Model file for the job. Use its own axes, mm. Face numbers are marked on the shaded views. Coordinates: 2 decimals unless noted, no trailing zeros. Write each loop counter-clockwise with the first axis right and the second up, starting at its lowest first coordinate (ties: lowest second). Pieces come first, ordered by that corner, then holes.
Q1. Pull direction Z, two halves, no side cores. Call the marked faces 1 and 2: released by +Z, released by -Z, zero draft, split by the parting line, or undercut.
Q2. Band-saw the part on C-C, the plane x = 46. Write the cut outline in (y, z), plus the area to 3 significant figures.
Q3. Drill centre lines: probe 1 along Z at (x, y) = (26, -1.55); probe 2 along Z at (x, y) = (-50, 0.8); probe 3 along Z at (x, y) = (58.4, 1.6). Where is each one in solid material? Low to high.
Q4. Pin check, flat tips, straight feed: P1, Ø1.1, axis at y = 1, z = 6.5, coming from the -X side; P2, Ø3, axis at x = 15.5, y = 2.5, coming from the -Z side; P3, Ø1, axis at x = -24, y = 1, coming from the +Z side. Stop position of each tip, or through.
Q5. Band-saw the part on D-D, the plane z = 2.1. Write the cut outline in (x, y).
Q6. Band-saw the part on A-A, the plane z = 9.2. Write the cut outline in (x, y), plus the area to 3 significant figures.
Q7. Band-saw the part on B-B, the plane x = -38. Write the cut outline in (y, z), plus the area to 3 significant figures.
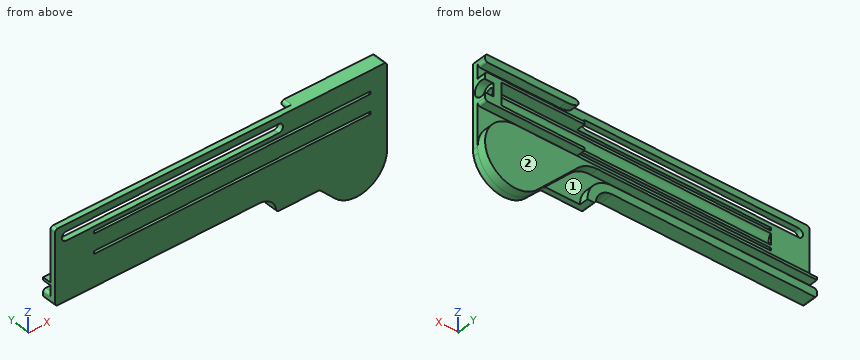
from build123d import *

# Parameters (mm, degrees)
BOSS_EXTRUDE2_DEPTH = 2
BOSS_EXTRUDE3_DEPTH = 3.2
BOSS_EXTRUDE4_START = 3.2
BOSS_EXTRUDE4_DEPTH = 3.2
SKETCH9_W           = 10
SKETCH9_H           = 3.2
BOSS_EXTRUDE5_DEPTH = 6
SKETCH8_R           = 2.8
CUT_EXTRUDE1_DEPTH  = 3.1
SKETCH10_R          = 1.4
CUT_EXTRUDE2_DEPTH  = 121.272440734
SKETCH11_R          = 2.55
CUT_EXTRUDE3_DEPTH  = 100
SKETCH12_W          = 30
SKETCH12_H          = 1
BOSS_EXTRUDE6_DEPTH = 3.2
SKETCH13_W          = 100
SKETCH13_H          = 1
CUT_EXTRUDE4_DEPTH  = 67.33136513
BOSS_EXTRUDE7_DEPTH = 3.2
CUT_EXTRUDE5_DEPTH  = 67.33136513
FILLET1_R           = 10
BOSS_EXTRUDE8_START = 2
BOSS_EXTRUDE8_DEPTH = 2
CUT_EXTRUDE6_DEPTH  = 67.33136513
FILLET2_R           = 1


with BuildPart() as part:
    # Sketch4 → Boss-Extrude2 (new body)
    with BuildSketch(Plane(origin=(0, 0, 0), x_dir=(1, 0, 0), z_dir=(0, 1, 0))):
        with BuildLine():
            Line((-60, -13.3), (60, -13.3))
            Line((60, -13.3), (60, 19.3))
            Line((60, 19.3), (20, 19.3))
            ThreePointArc((20, 19.3), (18.242640687, 15.057359313), (14, 13.3))
            Line((14, 13.3), (-60, 13.3))
            Line((-60, 13.3), (-60, -13.3))
        make_face()
    extrude(amount=-BOSS_EXTRUDE2_DEPTH)

    # Sketch5 → Boss-Extrude3 (add)
    with BuildSketch(Plane(origin=(0, 0, 0), x_dir=(1, 0, 0), z_dir=(0, 1, 0))):
        with BuildLine():
            Line((23.443650814, 7.1), (41.221825407, 24.878174593))
            ThreePointArc((41.221825407, 24.878174593), (59.162674858, 21.309517756), (49, 6.1))
            Line((49, 6.1), (-60, 6.1))
            Line((-60, 6.1), (-60, 7.1))
            Line((-60, 7.1), (23.443650814, 7.1))
        make_face()
    extrude(amount=BOSS_EXTRUDE3_DEPTH)

    # Sketch6 → Boss-Extrude4 (add)
    with BuildSketch(Plane(origin=(0, 0, 0), x_dir=(1, 0, 0), z_dir=(0, 1, 0)).offset(BOSS_EXTRUDE4_START)):
        with BuildLine():
            Line((-60, 10.3), (14, 10.3))
            ThreePointArc((14, 10.3), (20.363961031, 12.936038969), (23, 19.3))
            Line((23, 19.3), (20, 19.3))
            ThreePointArc((20, 19.3), (18.242640687, 15.057359313), (14, 13.3))
            Line((14, 13.3), (-60, 13.3))
            Line((-60, 13.3), (-60, 10.3))
        make_face()
    extrude(amount=-BOSS_EXTRUDE4_DEPTH)

    # Sketch9 → Boss-Extrude5 (add)
    with BuildSketch(Plane(origin=(60, 0, 0), x_dir=(0, 0, -1), z_dir=(1, 0, 0))):
        with Locations((-2.1, 1.6)):
            Rectangle(SKETCH9_W, SKETCH9_H)
    extrude(amount=-BOSS_EXTRUDE5_DEPTH)

    # Sketch8 → Cut-Extrude1 (cut)
    with BuildSketch(Plane(origin=(60, 0, 0), x_dir=(0, 0, -1), z_dir=(1, 0, 0))):
        with Locations((-2.1, 1.6)):
            Circle(SKETCH8_R)
    extrude(amount=-CUT_EXTRUDE1_DEPTH, mode=Mode.SUBTRACT)

    # Sketch10 → Cut-Extrude2 (cut, through all)
    with BuildSketch(Plane(origin=(56.9, 0, 0), x_dir=(0, 0, -1), z_dir=(1, 0, 0))):
        with Locations((-2.1, 1.6)):
            Circle(SKETCH10_R)
    extrude(amount=-CUT_EXTRUDE2_DEPTH, mode=Mode.SUBTRACT)

    # Sketch11 → Cut-Extrude3 (cut)
    with BuildSketch(Plane.ZY.offset(-54)):
        with Locations((2.1, 1.6)):
            Circle(SKETCH11_R)
    extrude(amount=CUT_EXTRUDE3_DEPTH, mode=Mode.SUBTRACT)

    # Sketch12 → Boss-Extrude6 (add)
    with BuildSketch(Plane(origin=(0, 0, 0), x_dir=(1, 0, 0), z_dir=(0, 1, 0))):
        with Locations((39, 2.4)):
            Rectangle(SKETCH12_W, SKETCH12_H)
    boss_extrude6 = extrude(amount=BOSS_EXTRUDE6_DEPTH)

    # Sketch13 → Cut-Extrude4 (cut, through all)
    with BuildSketch(Plane(origin=(0, 0, 0), x_dir=(1, 0, 0), z_dir=(0, 1, 0))):
        with Locations((4, 1.4)):
            Rectangle(SKETCH13_W, SKETCH13_H)
    cut_extrude4 = extrude(amount=-CUT_EXTRUDE4_DEPTH, mode=Mode.SUBTRACT)

    # Mirror1: Boss-Extrude6, Cut-Extrude4 across plane
    add(boss_extrude6.mirror(Plane.XY.offset(2.1)))
    add(cut_extrude4.mirror(Plane.XY.offset(2.1)), mode=Mode.SUBTRACT)

    # Sketch14 → Boss-Extrude7 (add)
    with BuildSketch(Plane(origin=(0, 0, 0), x_dir=(1, 0, 0), z_dir=(0, 1, 0))):
        with BuildLine():
            Line((60, -10.6), (30.518376618, -10.6))
            ThreePointArc((30.518376618, -10.6), (26.990656613, -11.301707138), (24, -13.3))
            Line((24, -13.3), (60, -13.3))
            Line((60, -13.3), (60, -10.6))
        make_face()
    extrude(amount=BOSS_EXTRUDE7_DEPTH)

    # Sketch15 → Cut-Extrude5 (cut, through all)
    with BuildSketch(Plane(origin=(0, 0, 0), x_dir=(1, 0, 0), z_dir=(0, 1, 0))):
        with BuildLine():
            Line((-56, -7.6), (20.8, -7.6))
            ThreePointArc((20.8, -7.6), (22.4, -9.2), (20.8, -10.8))
            Line((20.8, -10.8), (-56, -10.8))
            ThreePointArc((-56, -10.8), (-57.6, -9.2), (-56, -7.6))
        make_face()
    extrude(amount=-CUT_EXTRUDE5_DEPTH, mode=Mode.SUBTRACT)

    # Fillet1
    fillet1_edges = [part.edges().sort_by_distance(p)[0] for p in [
        (23.443650814, 1.6, -7.1),
    ]]
    fillet(fillet1_edges, radius=FILLET1_R)

    # Sketch16 → Boss-Extrude8 (add)
    with BuildSketch(Plane.XZ.offset(BOSS_EXTRUDE8_START)):
        with BuildLine():
            Line((59.777754868, -19.3), (35.643650814, -19.3))
            Line((35.643650814, -19.3), (41.221825407, -24.878174593))
            ThreePointArc((41.221825407, -24.878174593), (52.166761501, -27.634306887), (59.777754868, -19.3))
        make_face()
    extrude(amount=-BOSS_EXTRUDE8_DEPTH)

    # Sketch17 → Cut-Extrude6 (cut, through all)
    with BuildSketch(Plane(origin=(0, 0, 0), x_dir=(1, 0, 0), z_dir=(0, 1, 0))):
        with BuildLine():
            Line((60, 17.1), (60, 19.3))
            Line((60, 19.3), (59.777754868, 19.3))
            ThreePointArc((59.777754868, 19.3), (59.944297683, 18.205598582), (60, 17.1))
        make_face()
    extrude(amount=-CUT_EXTRUDE6_DEPTH, mode=Mode.SUBTRACT)

    # Fillet2
    fillet2_edges = [part.edges().sort_by_distance(p)[0] for p in [
        (-60, 0.6, -13.3),
        (20, 0.6, -19.3),
        (60, 0.6, 13.3),
        (-60, -1, 13.3),
        (60, 1.6, 10.6),
        (24, 1.6, 13.3),
        (35.643650814, -1, -19.3),
        (-60, 1.6, -10.3),
        (60, 1.6, -2.9),
        (60, 1.6, 7.1),
    ]]
    fillet(fillet2_edges, radius=FILLET2_R)


solid = part.part
Answer sheet:
1. face 1: undercut
1. face 2: zero draft
2. outline: (-2, -27.68) - (3.2, -27.68) - (3.2, -6.1) - (0, -6.1) - (0, -2.9) - (3.2, -2.9) - (3.2, -1.9) - (-2, -1.9) - close; (-2, -0.9) - (0, -0.9) - (0, 0.11) arc R2.55 cw to (0, 4.09) - (0, 5.1) - (-2, 5.1) - close; (-2, 6.1) - (3.2, 6.1) - (3.2, 7.1) - (0, 7.1) - (0, 10.6) - (3.2, 10.6) - (3.2, 13.3) - (-2, 13.3) - close
2. area: 159 mm2
3. probe 1: z = -19.3 to -1.9, -0.9 to 5.1, 6.1 to 13.3
3. probe 2: z = -13.3 to -10.3, -7.1 to -6.1
3. probe 3: z = -22.81 to -11.39, -2.9 to -0.7, 4.9 to 7.1, 10.6 to 13.3
4. P1: stops at x = 24
4. P2: stops at z = -14.1
4. P3: stops at z = -6.1
5. outline: (-60, -2) - (60, -2) - (60, -1.2) - (56.9, -1.2) - (56.9, 0.2) - (54, 0.2) - (54, -0.95) - (-46, -0.95) - (-46, 0) - (-60, 0) - close; (54, 3) - (56.9, 3) - (56.9, 3.2) - (54, 3.2) - close
6. outline: (-60, -2) - (-57.6, -2) - (-57.6, 0) - (-60, 0) - close; (22.4, -2) - (60, -2) - (60, 0) - (22.4, 0) - close
6. area: 80.0 mm2
7. outline: (-2, -13.3) - (3.2, -13.3) - (3.2, -10.3) - (0, -10.3) - (0, -7.1) - (3.2, -7.1) - (3.2, -6.1) - (0, -6.1) - (0, -1.9) - (-2, -1.9) - close; (-2, -0.9) - (0, -0.9) - (0, 0.11) arc R2.55 cw to (0, 4.09) - (0, 5.1) - (-2, 5.1) - close; (-2, 6.1) - (0, 6.1) - (0, 7.6) - (-2, 7.6) - close; (-2, 10.8) - (0, 10.8) - (0, 13.3) - (-2, 13.3) - close
7. area: 53.0 mm2
